from build123d import *

# Parameters (mm, degrees)
SKETCH1_W            = 25
SKETCH1_H            = 14
BOSS_EXTRUDE1_DEPTH  = 5
SKETCH2_W            = 25
SKETCH2_H            = 5
SKETCH2_H_2          = 15
BOSS_EXTRUDE2_DEPTH  = 3
M6_CLEARANCE_HOLE1_D = 6.6
SKETCH10_W           = 25
SKETCH10_H           = 5
BOSS_EXTRUDE5_DEPTH  = 2
SKETCH5_W            = 25
SKETCH5_H            = 5
BOSS_EXTRUDE4_DEPTH  = 40
CUT_EXTRUDE1_REACH   = 57.283
SKETCH9_R            = 1.5
FILLET1_R            = 2
BOSS_EXTRUDE6_DEPTH  = 3


with BuildPart() as part:
    # Sketch1 → Boss-Extrude1 (new body)
    with BuildSketch(Plane(origin=(0, 0, 0), x_dir=(1, 0, 0), z_dir=(0, 1, 0))):
        Rectangle(SKETCH1_W, SKETCH1_H)
    extrude(amount=BOSS_EXTRUDE1_DEPTH)

    # Sketch2 → Boss-Extrude2 (add)
    with BuildSketch(Plane.XY.offset(7)):
        with Locations((0, 2.5)):
            Rectangle(SKETCH2_W, SKETCH2_H)
        with Locations((0, -7.5)):
            Rectangle(SKETCH2_W, SKETCH2_H_2)
    extrude(amount=BOSS_EXTRUDE2_DEPTH)

    # M6 Clearance Hole1 (through all)
    with Locations(Plane.XY.offset(10)):
        with Locations((0, -6.5)):
            Hole(M6_CLEARANCE_HOLE1_D / 2)

    # Sketch10 → Boss-Extrude5 (add)
    with BuildSketch(Plane(origin=(0, 0, -7), x_dir=(-1, 0, 0), z_dir=(0, 0, -1))):
        Polygon((-12.5, 0), (-12.5, -3.2), (1e-09, -3.2), (12.5, -3.2), (12.5, 0), align=None)
        with Locations((0, 2.5)):
            Rectangle(SKETCH10_W, SKETCH10_H)
    extrude(amount=BOSS_EXTRUDE5_DEPTH)

    # Sketch5 → Boss-Extrude4 (add)
    with BuildSketch(Plane.XY.offset(10)):
        with Locations((0, 2.5)):
            Rectangle(SKETCH5_W, SKETCH5_H)
    extrude(amount=BOSS_EXTRUDE4_DEPTH)

    # Sketch9 → Cut-Extrude1 (cut, up to next)
    with BuildSketch(Plane(origin=(0, 5, 0), x_dir=(1, 0, 0), z_dir=(0, 1, 0)), mode=Mode.PRIVATE) as cut_extrude1_sk1:
        with Locations(Location((0, -41.5, 0), (0, 0, 270))):
            Circle(SKETCH9_R)
    cut_extrude1_tool1 = extrude(cut_extrude1_sk1.sketch, amount=-CUT_EXTRUDE1_REACH, mode=Mode.PRIVATE) & part.part
    add(cut_extrude1_tool1.solids().sort_by_distance((0, 5, 41.5))[0], mode=Mode.SUBTRACT)

    # Fillet1
    fillet1_edges = [part.edges().sort_by_distance(p)[0] for p in [
        (12.5, 0, 30),
        (-12.5, 0, 30),
        (0, -15, 10),
        (0, -3.2, -9),
        (0, 5, -9),
        (12.5, 5, 20.5),
        (0, 0, 50),
        (0, 5, 50),
        (-12.5, 5, 20.5),
        (0, 0, 10),
        (12.5, -7.5, 10),
        (-12.5, -7.5, 10),
        (-12.5, 0.9, -9),
        (12.5, 0.9, -9),
        (-12.5, 2.5, 50),
        (12.5, 2.5, 50),
    ]]
    fillet(fillet1_edges, radius=FILLET1_R - 0.0001)  # a hair under: the kernel refuses the full size

    # Sketch11 → Boss-Extrude6 (add)
    with BuildSketch(Plane.XZ):
        Polygon((4.5, 38.901923789), (4.5, 44.098076211), (0, 46.696152423), (-4.5, 44.098076211), (-4.5, 38.901923789), (0, 36.303847577), align=None)
        Polygon((0, 44.964101615), (-3, 43.232050808), (-3, 39.767949192), (0, 38.035898385), (3, 39.767949192), (3, 43.232050808), align=None, mode=Mode.SUBTRACT)
    extrude(amount=BOSS_EXTRUDE6_DEPTH)


solid = part.part
The model under review builds one solid part; all positions refer to its coordinate system, in mm. A direction names the side the tool comes from. Round coordinates to 2 decimals unless told otherwise and drop trailing zeros. Order: outer loops, then holes, each group sorted by start corner. A loop starts at its lowest first (then second) coordinate and runs counter-clockwise, first axis right, second up. Notation, with made-up numbers: (1, 30.5) - (36, 30.5) arc R13 cw to (36, 37.5) - close; hole circle Ø6 at (33, 20.5). An arc over 180 degrees is marked (long way). Use one line per item in the form item = value.
Q1. Add section D-D on z = 17. Give the boundary of the cut face in (x, y), then the cut area to 3 significant figures.
Response values:
outline = (-12.5, 2) arc R2 ccw to (-10.5, 0) - (10.5, 0) arc R2 ccw to (12.5, 2) - (12.5, 3) arc R2 ccw to (10.5, 5) - (-10.5, 5) arc R2 ccw to (-12.5, 3) - close
area = 122 mm^2
Q2. Add section B-B on z = 41.5. Give the boundary of the cut face in (x, y).
Response values:
outline = (-12.5, 2) arc R2 ccw to (-10.5, 0) - (-4.5, 0) - (-4.5, -3) - (-3, -3) - (-3, 0) - (-1.5, 0) - (-1.5, 5) - (-10.5, 5) arc R2 ccw to (-12.5, 3) - close; (1.5, 0) - (3, 0) - (3, -3) - (4.5, -3) - (4.5, 0) - (10.5, 0) arc R2 ccw to (12.5, 2) - (12.5, 3) arc R2 ccw to (10.5, 5) - (1.5, 5) - close
Q3. Tool access review of faces 1 (the flat face through (-1.5, -1.5, 38.9)), 2 (the cylindrical face through (-0.17, -2.6, -8.43)), 3 (the flat face through (0, -2, -7)), 4 (the cylindrical face through (0, 3, 40)), 5 (the cylindrical face through (11.9, 0.57, 30.25)): name each direction out of +Z, -Z, +X, -X, +Y, -Y from which nothing blocks a thin tool from reaching the whole face with its end or side.
Response values:
face_1 = -Y
face_2 = -Z, +X, -X, -Y
face_3 = +X, -X, -Y
face_4 = +Y, -Y
face_5 = +Z, +X, -Y
Q4. Clearance check with flat-ended pins moving along their axes: P1, Ø7.5, axis at x = 0, y = -6.5, coming from the +Z side; P2, Ø3.5, axis at y = -1, z = 42.5, coming from the +X side; P3, Ø2.5, axis at y = -2, z = 41, coming from the +X side; P4, Ø5, axis at y = -12, z = 14, coming from the +X side. State where each tip first meets the part, or that it passes through.
Response values:
P1 = 46.7
P2 = 12.06
P3 = 4.5
P4 = through
Q5. Add section A-A on y = -6.5. Give the boundary of the cut face in (x, z), then the cut area to 3 significant figures.
Response values:
outline = (-12.5, 7) - (-3.3, 7) - (-3.3, 10) - (-10.5, 10) arc R2 ccw to (-12.5, 8) - close; (3.3, 7) - (12.5, 7) - (12.5, 8) arc R2 ccw to (10.5, 10) - (3.3, 10) - close
area = 53.5 mm^2
Q6. Mouldability with a two-part tool opening along X and no side actions: class faces 6 (the flat face through (-1.5, -1.5, 44.1)), 7 (the flat face through (-2.218, -1.479, 45.415)), 8 (the flat face through (3, -1, 41)), 9 (the cylindrical face through (0.15, 4.4, 49.43)) as pulls with the +X half, pulls with the -X half, needs draft (parallel to the pull), parting line crosses it, or undercut.
Response values:
face_6 = undercut
face_7 = pulls with the -X half
face_8 = undercut
face_9 = needs draft
Q7. To check wall thickness, follow line 1 (Y direction, x = -2.75, z = 13.5); line 2 (Y direction, x = 1.25, z = 45.5); line 3 (Z direction, x = 1.75, y = -12.5). State the ranges of each line that lie inside material, in increasing order.
Response values:
line_1 = 0 to 5
line_2 = -3 to 5
line_3 = 7 to 10
